Build history of the part. All positions in model axes, mm. A direction names the side the tool comes from. Round coordinates to 2 decimals unless told otherwise and drop trailing zeros. Loops run counter-clockwise (first coordinate to the right, second up) from the corner with the lowest first, then second, coordinate; pieces in that order, holes last.
from build123d import *

# Parameters (mm, degrees)
SKETCH_1_R      = 12.25
SKETCH_1_R_2    = 1.6
EXTRUDE_1_DEPTH = 3
EXTRUDE_START   = 3
SKETCH_1_3_R    = 12.25
SKETCH_1_3_R_2  = 1.6
EXTRUDE_2_DEPTH = 3
SKETCH_1_4_R    = 1.6
EXTRUDE_3_DEPTH = 3
SKETCH_1_5_R    = 12.25
SKETCH_1_5_R_2  = 1.6
EXTRUDE_4_DEPTH = 3


with BuildPart() as part:
    # 草图1 → 凸台-拉伸1 (new body)
    # profile 1 of 2: a face of its own
    with BuildSketch(Plane(origin=(0, 0, 0), x_dir=(1, 0, 0), z_dir=(0, 1, 0))):
        with Locations(Location((0, 0, 0), (0, 0, 270))):
            Circle(SKETCH_1_R)
        with Locations(Location((-8, 0, 0), (0, 0, 270))):
            Circle(SKETCH_1_R_2, mode=Mode.SUBTRACT)
        with Locations(Location((0, -8, 0), (0, 0, 270))):
            Circle(SKETCH_1_R_2, mode=Mode.SUBTRACT)
        with Locations(Location((8, 0, 0), (0, 0, 270))):
            Circle(SKETCH_1_R_2, mode=Mode.SUBTRACT)
        with Locations(Location((0, 8, 0), (0, 0, 270))):
            Circle(SKETCH_1_R_2, mode=Mode.SUBTRACT)
        Polygon((-2.85, -1.645448267), (0, -3.290896534), (2.85, -1.645448267), (2.85, 1.645448267), (0, 3.290896534), (-2.85, 1.645448267), align=None, mode=Mode.SUBTRACT)
    # profile 2 of 2: a face of its own
    with BuildSketch(Plane(origin=(0, 0, 0), x_dir=(1, 0, 0), z_dir=(0, 1, 0))):
        Polygon((-2.85, 1.645448267), (-2.85, -1.645448267), (0, -3.290896534), (2.85, -1.645448267), (2.85, 1.645448267), (0, 3.290896534), align=None)
        with Locations(Location((0, 0, 0), (0, 0, 270))):
            Circle(SKETCH_1_R_2, mode=Mode.SUBTRACT)
    extrude(amount=-EXTRUDE_1_DEPTH)

    # 草图1<3> → 凸台-拉伸2 (add)
    with BuildSketch(Plane(origin=(0, 0, 0), x_dir=(1, 0, 0), z_dir=(0, 1, 0)).offset(EXTRUDE_START)):
        with Locations(Location((0, 0, 0), (0, 0, 270))):
            Circle(SKETCH_1_3_R)
        with Locations(Location((-8, 0, 0), (0, 0, 270))):
            Circle(SKETCH_1_3_R_2, mode=Mode.SUBTRACT)
        with Locations(Location((0, -8, 0), (0, 0, 270))):
            Circle(SKETCH_1_3_R_2, mode=Mode.SUBTRACT)
        with Locations(Location((8, 0, 0), (0, 0, 270))):
            Circle(SKETCH_1_3_R_2, mode=Mode.SUBTRACT)
        with Locations(Location((0, 8, 0), (0, 0, 270))):
            Circle(SKETCH_1_3_R_2, mode=Mode.SUBTRACT)
        Polygon((-2.85, -1.645448267), (0, -3.290896534), (2.85, -1.645448267), (2.85, 1.645448267), (0, 3.290896534), (-2.85, 1.645448267), align=None, mode=Mode.SUBTRACT)
    extrude(amount=-EXTRUDE_2_DEPTH)

    # 草图1<4> → 凸台-拉伸3 (add)
    with BuildSketch(Plane(origin=(0, 0, 0), x_dir=(1, 0, 0), z_dir=(0, 1, 0)).offset(EXTRUDE_START)):
        Polygon((-2.85, 1.645448267), (-2.85, -1.645448267), (0, -3.290896534), (2.85, -1.645448267), (2.85, 1.645448267), (0, 3.290896534), align=None)
        with Locations(Location((0, 0, 0), (0, 0, 270))):
            Circle(SKETCH_1_4_R, mode=Mode.SUBTRACT)
    extrude(amount=-EXTRUDE_3_DEPTH)

    # 草图1<5> → 凸台-拉伸4 (add)
    with BuildSketch(Plane(origin=(0, 0, 0), x_dir=(1, 0, 0), z_dir=(0, 1, 0)).offset(EXTRUDE_START)):
        with Locations(Location((0, 0, 0), (0, 0, 270))):
            Circle(SKETCH_1_5_R)
        with Locations(Location((-8, 0, 0), (0, 0, 270))):
            Circle(SKETCH_1_5_R_2, mode=Mode.SUBTRACT)
        with Locations(Location((0, -8, 0), (0, 0, 270))):
            Circle(SKETCH_1_5_R_2, mode=Mode.SUBTRACT)
        with Locations(Location((8, 0, 0), (0, 0, 270))):
            Circle(SKETCH_1_5_R_2, mode=Mode.SUBTRACT)
        with Locations(Location((0, 8, 0), (0, 0, 270))):
            Circle(SKETCH_1_5_R_2, mode=Mode.SUBTRACT)
        Polygon((-2.85, -1.645448267), (0, -3.290896534), (2.85, -1.645448267), (2.85, 1.645448267), (0, 3.290896534), (-2.85, 1.645448267), align=None, mode=Mode.SUBTRACT)
    extrude(amount=EXTRUDE_4_DEPTH)


solid = part.part
(1) Slice it at D-D on x = -8. List the corners of the cut face in (y, z), plus the area to 3 significant figures.
Responses:
outline: (-3, -9.28) - (6, -9.28) - (6, -1.6) - (-3, -1.6) - close; (-3, 1.6) - (6, 1.6) - (6, 9.28) - (-3, 9.28) - close
area: 138 mm2
(2) Probe line 1 (X direction, y = 4.15, z = 0); line 2 (X direction, y = 1.5, z = -0.25); line 3 (Z direction, x = -7, y = 0.5). List the from-to ranges inside material, lowest first.
Responses:
line 1: x = -12.25 to -9.6, -6.4 to -2.85, 2.85 to 6.4, 9.6 to 12.25
line 2: x = -12.25 to -9.58, -6.42 to -1.58, 1.58 to 6.42, 9.58 to 12.25
line 3: z = -10.05 to -1.25, 1.25 to 10.05
(3) Slice it at A-A on z = 0. List the corners of the cut face in (x, y).
Responses:
outline: (-12.25, -3) - (-9.6, -3) - (-9.6, 6) - (-12.25, 6) - close; (-6.4, -3) - (-1.6, -3) - (-1.6, 3) - (-2.85, 3) - (-2.85, 6) - (-6.4, 6) - close; (1.6, -3) - (6.4, -3) - (6.4, 6) - (2.85, 6) - (2.85, 3) - (1.6, 3) - close; (9.6, -3) - (12.25, -3) - (12.25, 6) - (9.6, 6) - close
(4) Pull direction X, two halves, no side cores. Call faces 3 (the face through (-3, 6, 3)), 4 (the face through (2.85, 4, 0)): +X half, -X half, draft (parallel to the pull), parting line (faces both ways), or undercut.
Responses:
face 3: draft
face 4: undercut
(5) Slice it at B-B on y = 0.25. List the corners of the cut face in (x, z).
Responses:
outline: circle Ø24.5 at (0, 0); hole circle Ø3.2 at (-8, 0); hole circle Ø3.2 at (0, -8); hole circle Ø3.2 at (0, 0); hole circle Ø3.2 at (0, 8); hole circle Ø3.2 at (8, 0)
(6) Which spindle directions (+Z, -Z, +X, -X, +Y, -Y) get a long thin tool onto all of the face, cutting with end or side? Do faces 1 (the face through (1, 3, -2)), 2 (the face through (-0.97, 0.04, -1.27)). Say none if no direction does.
Responses:
face 1: +Y
face 2: +Y, -Y
(7) Slice it at C-C on z = -7.75. List the corners of the cut face in (x, y), plus the area to 3 significant figures.
Responses:
outline: (-9.49, -3) - (-1.58, -3) - (-1.58, 6) - (-9.49, 6) - close; (1.58, -3) - (9.49, -3) - (9.49, 6) - (1.58, 6) - close
area: 142 mm2
(8) Pin check, flat tips, straight feed: P1, Ø1.5, axis at x = -9, y = 2.5, coming from the +Z side; P2, Ø1.5, axis at y = 5, z = 7.5, coming from the +X side; P3, Ø3.5, axis at x = -8, z = 0, coming from the +Y side; P4, Ø3, axis at x = 0, z = 0, coming from the -Y side. Stop position of each tip, or through.
Responses:
P1: stops at z = 9.06
P2: stops at x = 10.22
P3: stops at y = 6
P4: passes through
